Print and shaded views of the part. All mm, measured from the part's lowest x, y and z. A direction names the side the tool comes from. Give positions to 0.01 mm unless a question says otherwise; leave off trailing zeros. Loops run counter-clockwise (first coordinate to the right, second up) from the corner with the lowest first, then second, coordinate; pieces in that order, holes last.
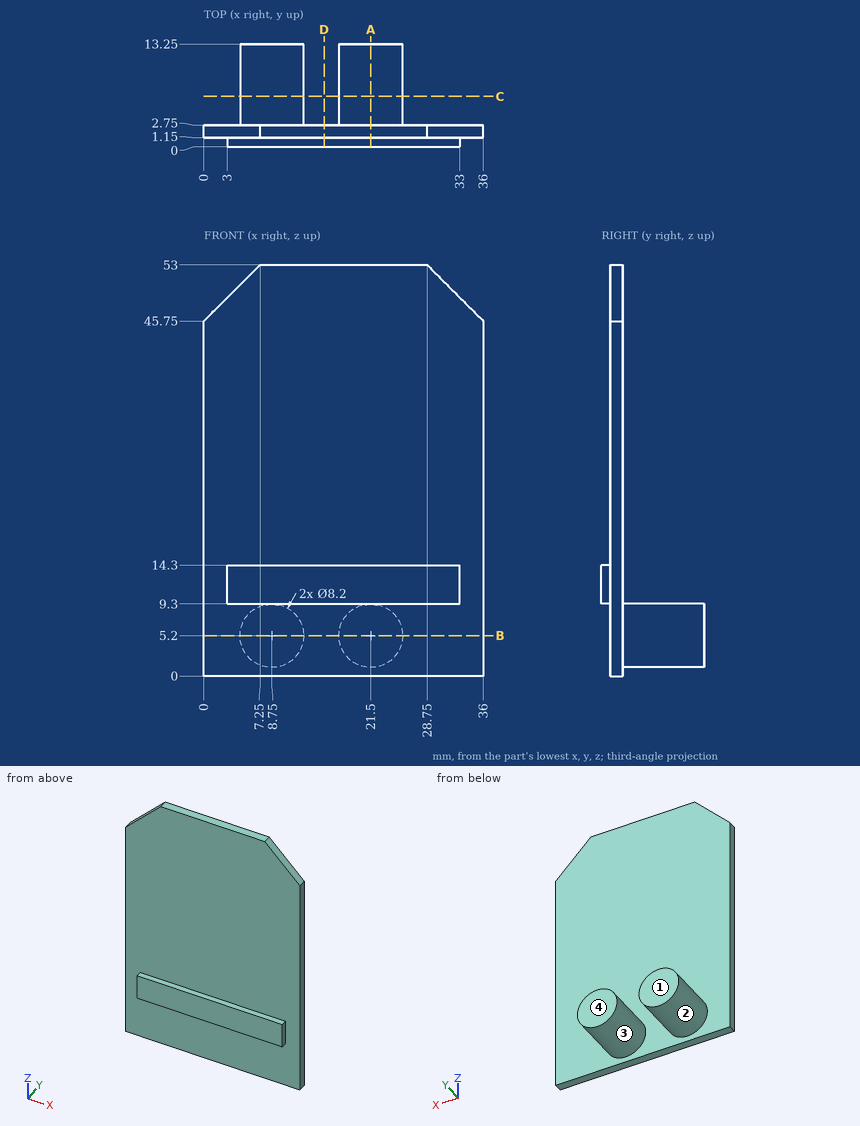
1. Saw through at D-D, the plane x = 15.5. List the corners of the cut face in (y, z).
Responses:
outline: (0, 9.3) - (1.15, 9.3) - (1.15, 0) - (2.75, 0) - (2.75, 53) - (1.15, 53) - (1.15, 14.3) - (0, 14.3) - close
2. Drop flat-ended pins along their axis: pin 1 (11 mm diameter, centred on x = 18, z = 22, fed in from +Y); pin 2 (8 mm diameter, centred on x = 26.5, z = 38, fed in from -Y); pin 3 (0.9 mm diameter, centred on x = 15, y = 0.5, fed in from -Z). Give the stop position or say it passes through.
Responses:
pin 1: stops at y = 2.75
pin 2: stops at y = 1.15
pin 3: stops at z = 9.3
3. Saw through at B-B, the plane z = 5.2. List the corners of the cut face in (x, y).
Responses:
outline: (0, 1.15) - (36, 1.15) - (36, 2.75) - (25.6, 2.75) - (25.6, 13.25) - (17.4, 13.25) - (17.4, 2.75) - (12.85, 2.75) - (12.85, 13.25) - (4.65, 13.25) - (4.65, 2.75) - (0, 2.75) - close
4. Probe line 1 along Y through (x, z) = (22, 43); line 2 along X through (y, z) = (11.25, 7); line 3 along Y through (x, z) = (10.5, 11). List the from-to ranges inside material, lowest first.
Responses:
line 1: y = 1.15 to 2.75
line 2: x = 5.07 to 12.43, 17.82 to 25.18
line 3: y = 0 to 2.75
5. Pull direction X, two halves, no side cores. Call the marked faces 1 and 2: released by +X, released by -X, zero draft, split by the parting line, or undercut.
Responses:
face 1: zero draft
face 2: undercut
6. Saw through at C-C, the plane y = 6.5. List the corners of the cut face in (x, z).
Responses:
outline: circle Ø8.2 at (8.75, 5.2); circle Ø8.2 at (21.5, 5.2)
7. Tool access for the marked faces 3 and 4: list every direction of +Z, -Z, +X, -X, +Y, -Y with a clear straight run to the whole face (end or side of a thin tool).
Responses:
face 3: +Y
face 4: +Z, -Z, +X, -X, +Y
8. Saw through at A-A, the plane x = 21.5. List the corners of the cut face in (y, z), and give its area (3 significant figures).
Responses:
outline: (0, 9.3) - (1.15, 9.3) - (1.15, 0) - (2.75, 0) - (2.75, 1.1) - (13.25, 1.1) - (13.25, 9.3) - (2.75, 9.3) - (2.75, 53) - (1.15, 53) - (1.15, 14.3) - (0, 14.3) - close
area: 177 mm2
